Can you work these out from the model? Positions are in its coordinate system, mm. Coordinates: 2 decimals unless noted, no trailing zeros. Order: outer loops, then holes, each group sorted by start corner. A loop starts at its lowest first (then second) coordinate and runs counter-clockwise, first axis right, second up. Notation, with made-up numbers: (61.25, -40) -> (94.25, -40) arc R22 cw to (94.25, -13) -> close; hole circle Ø1 at (37, 58.5). An arc over 180 degrees is marked (long way). Answer in a Markdown table with one row per item. Add a question column.
1. Imagine slicing it at C-C on z = -189.5. Write out the boundary of the cut face in (x, y), plus the area to 3 significant figures.
2. If I drill on line 1 along Z through (x, y) = (240, 0.9); line 2 along X through (y, z) = (2.7, -66); line 3 along X through (y, z) = (2.65, -166), over which ranges is the centre line in solid material (lowest first)? Write a range as [from, to].
3. Imagine slicing it at D-D on x = 447.5. Write out the boundary of the cut face in (y, z), plus the area to 3 significant figures.
4. Imagine slicing it at B-B on y = 2.45. State how many separate pieces and enclosed holes the cut face has, plus the area to 3 significant figures.
5. Imagine slicing it at A-A on z = -117. Write out the boundary of the cut face in (x, y).
6. We'd pull the mould along Z, two halves only. Please class faces 1 (the face through (261, 3.5, -117)), 2 (the face through (482.214, 1.726, -118.951)): pulls with the +Z half, pulls with the -Z half, needs draft (parallel to the pull), parting line crosses it, or undercut.
7. Will this pin go through, and if not, where does the flat tip stop? pin 1 (1.8 mm diameter, centred on x = 491, y = 2, fed in from -Z).
from build123d import *

# Parameters (mm, degrees)
BOSS_EXTRUDE1_DEPTH     = 3.5
CUT_EXTRUDE1_DEPTH      = 565.036567963
CUT_EXTRUDE1_DEPTH_BACK = 565.036567963
SKETCH2_R               = 4
SKETCH2_R_2             = 9


with BuildPart() as part:
    # Sketch1 → Boss-Extrude1 (new body)
    with BuildSketch(Plane(origin=(0, 0, 0), x_dir=(1, 0, 0), z_dir=(0, 1, 0))):
        Polygon((0, 0), (0, 150), (0, 230), (20, 230), (439.5, 230), (439.5, 150), (515, 150), (515, 0), align=None)
    extrude(amount=BOSS_EXTRUDE1_DEPTH)

    # Sketch2 → Cut-Extrude1 (cut, two sides: drawn at the far end of the back side and taken through both)
    with BuildSketch(Plane(origin=(0, 3.5, 0), x_dir=(1, 0, 0), z_dir=(0, 1, 0)).offset(-CUT_EXTRUDE1_DEPTH_BACK)):
        with Locations(Location((115, 166, 0), (0, 0, 270))):
            Circle(SKETCH2_R)
        with Locations(Location((240, 166, 0), (0, 0, 270))):
            Circle(SKETCH2_R)
        with Locations(Location((365, 166, 0), (0, 0, 270))):
            Circle(SKETCH2_R)
        with Locations(Location((365, 66, 0), (0, 0, 270))):
            Circle(SKETCH2_R)
        with Locations(Location((240, 66, 0), (0, 0, 270))):
            Circle(SKETCH2_R)
        with Locations(Location((115, 66, 0), (0, 0, 270))):
            Circle(SKETCH2_R)
        with Locations(Location((492.517503026, 92.046098811, 0), (0, 0, 270))):
            Circle(SKETCH2_R_2)
        with Locations(Location((491, 117, 0), (0, 0, 270))):
            Circle(SKETCH2_R_2)
    extrude(amount=CUT_EXTRUDE1_DEPTH + CUT_EXTRUDE1_DEPTH_BACK, mode=Mode.SUBTRACT)


solid = part.part
Answers follow:
| question | item | result |
|---|---|---|
| 1 | outline | (0, 0) -> (439.5, 0) -> (439.5, 3.5) -> (0, 3.5) -> close |
| 1 | area | 1,540 mm² |
| 2 | line 1 | z = [-230, -170], [-162, -70], [-62, 0] |
| 2 | line 2 | x = [0, 111], [119, 236], [244, 361], [369, 515] |
| 2 | line 3 | x = [0, 111], [119, 236], [244, 361], [369, 439.5] |
| 3 | outline | (0, -150) -> (3.5, -150) -> (3.5, 0) -> (0, 0) -> close |
| 3 | area | 525 mm² |
| 4 | separate pieces | 1 |
| 4 | enclosed holes | 8 |
| 4 | area | 112,000 mm² |
| 5 | outline | (0, 0) -> (482, 0) -> (482, 3.5) -> (0, 3.5) -> close; (500, 0) -> (515, 0) -> (515, 3.5) -> (500, 3.5) -> close |
| 6 | face 1 | needs draft |
| 6 | face 2 | undercut |
| 7 | pin 1 | stops at z = -150 |
